```python
from build123d import *

# Parameters (mm, degrees)
SKETCH1_W           = 240
SKETCH1_H           = 60
BOSS_EXTRUDE1_DEPTH = 5
SKETCH2_W           = 235
SKETCH2_H           = 5
BOSS_EXTRUDE2_DEPTH = 88
BOSS_EXTRUDE3_START = 93
SKETCH1_2_W         = 240
SKETCH1_2_H         = 60
BOSS_EXTRUDE3_DEPTH = 5


with BuildPart() as part:
    # Sketch1 → Boss-Extrude1 (new body)
    with BuildSketch(Plane(origin=(0, 0, 0), x_dir=(1, 0, 0), z_dir=(0, 1, 0))):
        Rectangle(SKETCH1_W, SKETCH1_H)
    extrude(amount=BOSS_EXTRUDE1_DEPTH)

    # Sketch2 → Boss-Extrude2 (add)
    with BuildSketch(Plane(origin=(0, 5, 0), x_dir=(1, 0, 0), z_dir=(0, 1, 0))):
        with Locations((2.5, -27.5)):
            Rectangle(SKETCH2_W, SKETCH2_H)
        Polygon((-115, 30), (-120, 30), (-120, -30), (-115, -30), (-115, -25), (-115, 25), align=None)
        with Locations((2.5, 27.5)):
            Rectangle(SKETCH2_W, SKETCH2_H)
    extrude(amount=BOSS_EXTRUDE2_DEPTH)

    # Sketch1_2 → Boss-Extrude3 (add)
    with BuildSketch(Plane(origin=(0, 0, 0), x_dir=(1, 0, 0), z_dir=(0, 1, 0)).offset(BOSS_EXTRUDE3_START)):
        Rectangle(SKETCH1_2_W, SKETCH1_2_H)
    extrude(amount=BOSS_EXTRUDE3_DEPTH)


solid = part.part
```
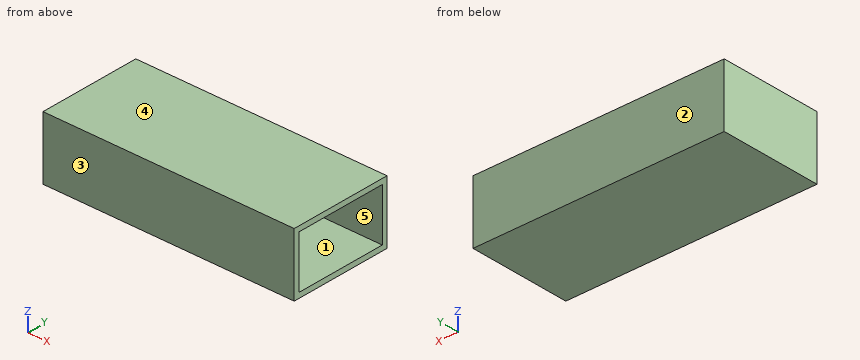
Source: CAD feature listing. Evaluate the final solid. Frame: model axes, mm. Face numbers are marked on the shaded views. A direction names the side the tool comes from. Coordinates: 2 decimals unless noted, no trailing zeros. Loops run counter-clockwise (first coordinate to the right, second up) from the corner with the lowest first, then second, coordinate; pieces in that order, holes last. Notation, with made-up numbers: (2.25, -0.5) -> (45.25, -0.5) arc R14 cw to (45.25, 17.5) -> close; hole circle Ø2 at (-15.5, -34.75). An arc over 180 degrees is marked (long way). One line per item, written item: value. Start each with the question number.
Q1. Set-up query: the marked faces 1 and 2. Return all of +Z, -Z, +X, -X, +Y, -Y with unobstructed straight access to the full face (end or side cutting, diameter ignored); none if empty.
Q2. Contact query for flat-ended pins moving along their axis: P1, Ø1.5, axis at x = -26.5, z = -13.5, coming from the -Y side; P2, Ø12, axis at y = 70, z = -15, coming from the +X side. Output: stop coordinate, or through.
Q3. Line query: line 1 along Z through (x, y) = (68, 31); line 2 along Y through (x, z) = (-74, -5); line 3 along X through (y, z) = (13.5, 12). Output: solid intervals per line, ascending.
Q4. Section query A-A, the plane x = -97.5. Return the cut outline in (y, z), and give its area (3 significant figures).
Q5. Mould query, pull axis Z, two halves, no side actions, for the marked faces 3, 4 and 5. Classes: pulls with the +Z half, pulls with the -Z half, needs draft (parallel to the pull), parting line crosses it, or undercut.
Q6. Section query C-C, the plane z = 8. Return the cut outline in (x, y), and give its area (3 significant figures).
Q7. Section query B-B, the plane y = 70.5. Return the cut outline in (x, z).
Results:
1. face 1: +X
1. face 2: +Z, -Z, +X, -X, +Y
2. P1: y = 0
2. P2: x = -115
3. line 1: -30 to -25, 25 to 30
3. line 2: 0 to 5, 93 to 98
3. line 3: -120 to -115
4. outline: (0, -30) -> (98, -30) -> (98, 30) -> (0, 30) -> close; hole (5, -25) -> (93, -25) -> (93, 25) -> (5, 25) -> close
4. area: 1,480 mm^2
5. face 3: needs draft
5. face 4: pulls with the +Z half
5. face 5: undercut
6. outline: (-120, 0) -> (120, 0) -> (120, 5) -> (-115, 5) -> (-115, 93) -> (120, 93) -> (120, 98) -> (-120, 98) -> close
6. area: 2,840 mm^2
7. outline: (-120, -30) -> (120, -30) -> (120, -25) -> (-115, -25) -> (-115, 25) -> (120, 25) -> (120, 30) -> (-120, 30) -> close
